Geometry: final body of the model. Coordinates: model frame, mm. Face numbers are marked on the shaded views. Give positions to 0.01 mm unless a question says otherwise; leave off trailing zeros. Write each loop counter-clockwise with the first axis right and the second up, starting at its lowest first coordinate (ties: lowest second). Pieces come first, ordered by that corner, then holes. Notation, with made-up numbers: (67.5, -26.75) -> (111.5, -26.75) arc R23 ccw to (111.5, 11.25) -> close; hole circle Ø8 at (73.25, 33.5). An arc over 180 degrees is marked (long way). Answer as a JSON object with one key per item and string values.
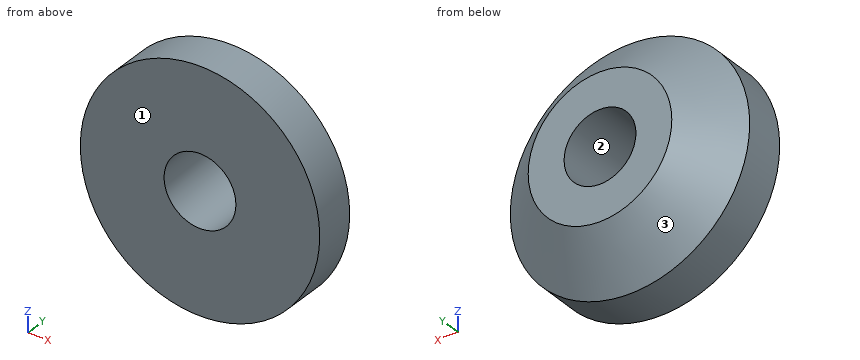
from build123d import *

# Parameters (mm, degrees)
SKETCH2_R           = 10
BOSS_EXTRUDE1_DEPTH = 3.5
SKETCH1_R           = 6
SKETCH3_R           = 3
CUT_EXTRUDE1_DEPTH  = 9.5


with BuildPart() as part:
    # Sketch2 → Boss-Extrude1 (new body)
    with BuildSketch(Plane(origin=(0, -7, 0), x_dir=(1, 0, 0), z_dir=(0, 1, 0))):
        Circle(SKETCH2_R)
    extrude(amount=BOSS_EXTRUDE1_DEPTH)

    # Sketch1 → section 0 of loft1
    with BuildSketch(Plane(origin=(0, 0, 0), x_dir=(1, 0, 0), z_dir=(0, 1, 0)), mode=Mode.PRIVATE) as loft1_s0:
        Circle(SKETCH1_R)
    # loft up to a face of the part (loft1)
    loft([loft1_s0.sketch, part.faces().sort_by_distance((0, -3.5, 0))[0]])

    # Sketch3 → Cut-Extrude1 (cut)
    with BuildSketch(Plane(origin=(0, 0, 0), x_dir=(1, 0, 0), z_dir=(0, 1, 0))):
        Circle(SKETCH3_R)
    extrude(amount=-CUT_EXTRUDE1_DEPTH, mode=Mode.SUBTRACT)


solid = part.part
Q1. First-contact query: P1, Ø1.5, axis at y = -2.5, z = 2, coming from the +X side; P2, Ø5, axis at x = 0, z = 0, coming from the +Y side; P3, Ø1.5, axis at y = -4, z = -7, coming from the +X side; P4, Ø3, axis at x = -6.5, y = -2, coming from the -Z side. Flat tips, straight axial feed; report the tip coordinate or a pass-through.
Values:
{"P1": "x = 9.52", "P2": "through", "P3": "x = 7.81", "P4": "z = -7.9"}
Q2. Cut plane C-C (y = -1.75). Return the cut outline in (x, z).
Values:
{"outline": "circle Ø16 at (0, 0); hole circle Ø6 at (0, 0)"}
Q3. Mould query, pull axis Z, two halves, no side actions, for the marked faces 1, 2 and 3. Classes: pulls with the +Z half, pulls with the -Z half, needs draft (parallel to the pull), parting line crosses it, or undercut.
Values:
{"face 1": "needs draft", "face 2": "undercut", "face 3": "parting line crosses it"}
Q4. Cut plane A-A (x = 0). Return the cut outline in (y, z).
Values:
{"outline": "(-7, -10) -> (-3.5, -10) -> (0, -6) -> (0, -3) -> (-7, -3) -> close; (-7, 3) -> (0, 3) -> (0, 6) -> (-3.5, 10) -> (-7, 10) -> close"}
Q5. Cut plane B-B (y = -4.5). Return the cut outline in (x, z), and give its area (3 significant figures).
Values:
{"outline": "circle Ø20 at (0, 0); hole circle Ø6 at (0, 0)", "area": "286 mm²"}
Q6. Material intervals for L1, parallel to X at y = -4, z = 0; L2, parallel to Z at x = 0, y = -3; L3, parallel to X at y = -1.25, z = 0, sorted ascending. Write a range as from..to.
Values:
{"L1": "-10..-3, 3..10", "L2": "-9.43..-3, 3..9.43", "L3": "-7.43..-3, 3..7.43"}
